from build123d import *

# Parameters (mm, degrees)
SKETCH1_W           = 150
SKETCH1_H           = 120
BODY_DEPTH          = 50
SPINE_SOCKET_DEPTH  = 151.083310198
SKETCH3_R           = 5
CUT_EXTRUDE2_DEPTH  = 47.5
SKETCH4_W           = 15
SKETCH4_H           = 120
SKETCH4_W_2         = 5
SKETCH4_H_2         = 110
BOSS_EXTRUDE2_DEPTH = 10


with BuildPart() as part:
    # Sketch1 → body (new body)
    with BuildSketch(Plane.XY):
        with Locations((0, 60)):
            Rectangle(SKETCH1_W, SKETCH1_H)
    extrude(amount=BODY_DEPTH)

    # Sketch2 → spine socket (cut, through all)
    with BuildSketch(Plane(origin=(0, 120, 0), x_dir=(1, 0, 0), z_dir=(0, 1, 0))):
        Polygon((-65, -5), (-65, -15), (-55, -15), (-55, -35), (-65, -35), (-65, -45), (65, -45), (65, -35), (55, -35), (55, -15), (65, -15), (65, -5), align=None)
    extrude(amount=-SPINE_SOCKET_DEPTH, mode=Mode.SUBTRACT)

    # Sketch3 → Cut-Extrude2 (cut)
    with BuildSketch(Plane.XY.offset(50)):
        with Locations((0, 110)):
            Circle(SKETCH3_R)
        with Locations((0, 80)):
            Circle(SKETCH3_R)
    extrude(amount=-CUT_EXTRUDE2_DEPTH, mode=Mode.SUBTRACT)

    # Sketch4 → Boss-Extrude2 (add)
    # profile 1 of 2: a face of its own
    with BuildSketch(Plane(origin=(0, 0, 0), x_dir=(-1, 0, 0), z_dir=(0, 0, -1))):
        with Locations((-82.5, 60)):
            Rectangle(SKETCH4_W, SKETCH4_H)
        with Locations((-82.5, 60)):
            Rectangle(SKETCH4_W_2, SKETCH4_H_2, mode=Mode.SUBTRACT)
    # profile 2 of 2: a face of its own
    with BuildSketch(Plane(origin=(0, 0, 0), x_dir=(-1, 0, 0), z_dir=(0, 0, -1))):
        with Locations((82.5, 60)):
            Rectangle(SKETCH4_W, SKETCH4_H)
        with Locations((82.5, 60)):
            Rectangle(SKETCH4_W_2, SKETCH4_H_2, mode=Mode.SUBTRACT)
    extrude(amount=-BOSS_EXTRUDE2_DEPTH)


solid = part.part
Input: part model. Units: mm. Frame: model coordinates. A direction names the side the tool comes from. Give positions to 0.01 mm unless a question says otherwise; leave off trailing zeros. Loops run counter-clockwise (first coordinate to the right, second up) from the corner with the lowest first, then second, coordinate; pieces in that order, holes last. Notation, with made-up numbers: M 12.5,18 L 50.5,18 A21 ccw 50.5,24 Z; hole C 63.5,22 d7. An arc over 180 degrees is marked long. Use CSV: the item, a comma, the result in double quotes.
(1) Pin query (flat end, axial travel): P1, Ø12, axis at y = 40.5, z = 37, coming from the -X side; P2, Ø7.5, axis at x = -81.5, y = 49, coming from the +Z side; P3, Ø6, axis at x = 0, y = 110, coming from the +Z side. Return the tip coordinate at first contact, or that it passes through.
Outcome:
P1,"stops at x = -75"
P2,"stops at z = 10"
P3,"stops at z = 2.5"
(2) Section A-A, the plane y = 100.5. Return loops of the section in (x, z), plus the area to 3 significant figures.
Outcome:
outline,"M -90,0 L -85,0 L -85,10 L -90,10 Z; M -80,0 L 80,0 L 80,10 L 75,10 L 75,50 L -75,50 L -75,10 L -80,10 Z; M 85,0 L 90,0 L 90,10 L 85,10 Z; hole M -65,5 L 65,5 L 65,15 L 55,15 L 55,35 L 65,35 L 65,45 L -65,45 L -65,35 L -55,35 L -55,15 L -65,15 Z"
area,"2,900 mm²"
(3) Section D-D, the plane x = 0. Return loops of the section in (y, z), plus the area to 3 significant figures.
Outcome:
outline,"M 0,0 L 120,0 L 120,5 L 115,5 L 115,2.5 L 105,2.5 L 105,5 L 85,5 L 85,2.5 L 75,2.5 L 75,5 L 0,5 Z; M 0,45 L 75,45 L 75,50 L 0,50 Z; M 85,45 L 105,45 L 105,50 L 85,50 Z; M 115,45 L 120,45 L 120,50 L 115,50 Z"
area,"1,050 mm²"
(4) Section C-C, the plane z = 18. Return loops of the section in (x, y).
Outcome:
outline,"M -75,0 L -55,0 L -55,120 L -75,120 Z; M 55,0 L 75,0 L 75,120 L 55,120 Z"
(5) Pull-direction query (X, two-part tool) for faces 6 (the face through (-79, 61, 10)), 7 (the face through (-1.08, 105.12, 3.77)), 8 (the face through (-75, 59, 30)); classes: pulls with the +X half, pulls with the -X half, needs draft (parallel to the pull), parting line crosses it, or undercut.
Outcome:
face 6,"needs draft"
face 7,"undercut"
face 8,"pulls with the -X half"
(6) Set-up query: faces 1 (the face through (-1.08, 105.12, 47.54)), 2 (the face through (1, 61, 5)), 3 (the face through (83, 5, 5)), 4 (the face through (90, 59, 5)), 5 (the face through (75, 59, 30)). Return all of +Z, -Z, +X, -X, +Y, -Y with unobstructed straight access to the full face (end or side cutting, diameter ignored); none if empty.
Outcome:
face 1,"+Z"
face 2,"+Y, -Y"
face 3,"+Z, -Z"
face 4,"+Z, -Z, +X, +Y, -Y"
face 5,"+Z, +X, +Y, -Y"
(7) Section B-B, the plane x = 23.5. Return loops of the section in (y, z).
Outcome:
outline,"M 0,0 L 120,0 L 120,5 L 0,5 Z; M 0,45 L 120,45 L 120,50 L 0,50 Z"
(8) Material intervals for L1, parallel to Z at x = -56, y = 96.5; L2, parallel to Y at x = 0, z = 3.95; L3, parallel to X at y = 15, z = 17, sorted ascending. Write a range as [from, to].
Outcome:
L1,"z = [0, 5], [15, 35], [45, 50]"
L2,"y = [0, 75], [85, 105], [115, 120]"
L3,"x = [-75, -55], [55, 75]"
